from build123d import *

# Parameters (mm, degrees)
CROQUIS1_W              = 8.5
CROQUIS1_H              = 10
SALIENTE_EXTRUIR1_DEPTH = 3.3
CROQUIS2_R              = 0.466725864
CORTAR_EXTRUIR1_DEPTH   = 0.1
CORTAR_EXTRUIR2_DEPTH   = 3
CORTAR_EXTRUIR3_DEPTH   = 3
CHAFL_N1_SIZE           = 0.6
REDONDEO1_R             = 0.3
CROQUIS5_W              = 8.5
CROQUIS5_H              = 0.8
SALIENTE_EXTRUIR2_DEPTH = 5.8
CROQUIS6_R              = 1.750484279
CORTAR_EXTRUIR4_DEPTH   = 5.8
CROQUIS7_W              = 1.22
CROQUIS7_H              = 0.3917794
SALIENTE_EXTRUIR3_DEPTH = 5.3
CROQUIS8_W              = 1.22
CROQUIS8_H              = 0.3917794
SALIENTE_EXTRUIR4_DEPTH = 5.3
CROQUIS9_W              = 0.675717965
CROQUIS9_H              = 1
CROQUIS9_W_2            = 0.619737604
CROQUIS9_W_3            = 0.713804918
SALIENTE_EXTRUIR5_DEPTH = 2.3
CHAFL_N2_SIZE           = 0.3
CHAFL_N3_SIZE           = 0.3
CHAFL_N4_SIZE           = 0.3
CHAFL_N5_SIZE           = 0.3
CHAFL_N6_SIZE           = 0.3
CHAFL_N7_SIZE           = 0.3
CHAFL_N8_SIZE           = 1.29
CHAFL_N9_SIZE           = 1.29


with BuildPart() as part:
    # Croquis1 → Saliente-Extruir1 (new body)
    with BuildSketch(Plane.XY):
        Rectangle(CROQUIS1_W, CROQUIS1_H)
    extrude(amount=SALIENTE_EXTRUIR1_DEPTH)

    # Croquis2 → Cortar-Extruir1 (cut)
    with BuildSketch(Plane.XY.offset(3.3)):
        with Locations((-3.215855375, -4.280210789)):
            Circle(CROQUIS2_R)
    extrude(amount=-CORTAR_EXTRUIR1_DEPTH, mode=Mode.SUBTRACT)

    # Croquis3 → Cortar-Extruir2 (cut)
    with BuildSketch(Plane.XY.offset(3.3)):
        with BuildLine():
            Line((-4.25, 0.746438526), (-4.25, -0.746438526))
            ThreePointArc((-4.25, -0.746438526), (-3.503561474, 0), (-4.25, 0.746438526))
        make_face()
    extrude(amount=-CORTAR_EXTRUIR2_DEPTH, mode=Mode.SUBTRACT)

    # Croquis4 → Cortar-Extruir3 (cut)
    with BuildSketch(Plane.XY.offset(3.3)):
        with BuildLine():
            Line((4.25, 0.878718771), (4.25, -0.633055459))
            ThreePointArc((4.25, -0.633055459), (3.494112885, 0.122831656), (4.25, 0.878718771))
        make_face()
    extrude(amount=-CORTAR_EXTRUIR3_DEPTH, mode=Mode.SUBTRACT)

    # Chaflán1
    chafl_n1_edges = [part.edges().sort_by_distance(p)[0] for p in [
        (0, 5, 3.3),
    ]]
    chamfer(chafl_n1_edges, length=CHAFL_N1_SIZE)

    # Redondeo1
    redondeo1_edges = [part.edges().sort_by_distance(p)[0] for p in [
        (4.25, -2.816527729, 3.3),
        (-4.25, -2.873219263, 3.3),
        (-3.503561474, 0, 3.3),
        (4.25, 2.639359386, 3.3),
        (3.494112885, 0.122831656, 3.3),
        (-4.25, 2.573219263, 3.3),
    ]]
    fillet(redondeo1_edges, radius=REDONDEO1_R)

    # Croquis5 → Saliente-Extruir2 (add)
    with BuildSketch(Plane(origin=(0, 5, 0), x_dir=(1, 0, 0), z_dir=(0, 1, 0))):
        with Locations((0, -0.4)):
            Rectangle(CROQUIS5_W, CROQUIS5_H)
    extrude(amount=SALIENTE_EXTRUIR2_DEPTH)

    # Croquis6 → Cortar-Extruir4 (cut)
    with BuildSketch(Plane.XY.offset(0.8)):
        with Locations((0, 8.041970686)):
            Circle(CROQUIS6_R)
    extrude(amount=-CORTAR_EXTRUIR4_DEPTH, mode=Mode.SUBTRACT)

    # Croquis7 → Saliente-Extruir3 (add)
    with BuildSketch(Plane.XZ.offset(5)):
        with Locations((0, 2.138324213)):
            Rectangle(CROQUIS7_W, CROQUIS7_H)
    extrude(amount=SALIENTE_EXTRUIR3_DEPTH)

    # Croquis8 → Saliente-Extruir4 (add)
    with BuildSketch(Plane.XZ.offset(5)):
        with Locations((2.43, 2.138324213)):
            Rectangle(CROQUIS8_W, CROQUIS8_H)
        with Locations((-2.43, 2.138324213)):
            Rectangle(CROQUIS8_W, CROQUIS8_H)
    extrude(amount=SALIENTE_EXTRUIR4_DEPTH)

    # Croquis9 → Saliente-Extruir5 (add)
    with BuildSketch(Plane(origin=(0, 0, 1.942434513), x_dir=(-1, 0, 0), z_dir=(0, 0, -1))):
        with Locations((-0.032858983, -9.8)):
            Rectangle(CROQUIS9_W, CROQUIS9_H)
        with Locations((2.407034508, -9.8)):
            Rectangle(CROQUIS9_W_2, CROQUIS9_H)
        with Locations((-2.448498949, -9.8)):
            Rectangle(CROQUIS9_W_3, CROQUIS9_H)
    extrude(amount=SALIENTE_EXTRUIR5_DEPTH)

    # Chaflán2
    chafl_n2_edges = [part.edges().sort_by_distance(p)[0] for p in [
        (3.04, -10.3, 2.138324213),
    ]]
    chamfer(chafl_n2_edges, length=CHAFL_N2_SIZE)

    # Chaflán3
    chafl_n3_edges = [part.edges().sort_by_distance(p)[0] for p in [
        (1.82, -10.3, 2.138324213),
    ]]
    chamfer(chafl_n3_edges, length=CHAFL_N3_SIZE)

    # Chaflán4
    chafl_n4_edges = [part.edges().sort_by_distance(p)[0] for p in [
        (-0.61, -10.3, 2.138324213),
    ]]
    chamfer(chafl_n4_edges, length=CHAFL_N4_SIZE)

    # Chaflán5
    chafl_n5_edges = [part.edges().sort_by_distance(p)[0] for p in [
        (-3.04, -10.3, 2.138324213),
    ]]
    chamfer(chafl_n5_edges, length=CHAFL_N5_SIZE)

    # Chaflán6
    chafl_n6_edges = [part.edges().sort_by_distance(p)[0] for p in [
        (-1.82, -10.3, 2.138324213),
    ]]
    chamfer(chafl_n6_edges, length=CHAFL_N6_SIZE)

    # Chaflán7
    chafl_n7_edges = [part.edges().sort_by_distance(p)[0] for p in [
        (0.61, -10.3, 2.138324213),
    ]]
    chamfer(chafl_n7_edges, length=CHAFL_N7_SIZE)

    # Chaflán8
    chafl_n8_edges = [part.edges().sort_by_distance(p)[0] for p in [
        (4.25, 10.8, 0.4),
    ]]
    chamfer(chafl_n8_edges, length=CHAFL_N8_SIZE)

    # Chaflán9
    chafl_n9_edges = [part.edges().sort_by_distance(p)[0] for p in [
        (-4.25, 10.8, 0.4),
    ]]
    chamfer(chafl_n9_edges, length=CHAFL_N9_SIZE)


solid = part.part
Source: CAD feature listing. Evaluate the final solid. Frame: model axes, mm. A direction names the side the tool comes from. Round coordinates to 2 decimals unless told otherwise and drop trailing zeros. Loops run counter-clockwise (first coordinate to the right, second up) from the corner with the lowest first, then second, coordinate; pieces in that order, holes last.
Q1. Section B-B, the plane x = 0. Return loops of the section in (y, z).
Q2. Access query for faces 1 (the face through (0, 6, 0.8)), 2 (the face through (0.371, -10, 1)), 3 (the face through (-3.504, -0.016, 1.669)). Directions: +Z, -Z, +X, -X, +Y, -Y. A direction counts if a zero-diameter tool reaches every point of the face in a straight line with its end or side. Return the directions, or none.
Q3. First-contact query: P1, Ø1, axis at x = 0, y = -8, coming from the -Z side; P2, Ø2.5, axis at x = 1, y = 0, coming from the -Z side; P3, Ø4, axis at x = 0, y = 8.04, coming from the +Z side. Flat tips, straight axial feed; report the tip coordinate or a pass-through.
Q4. Mould query, pull axis Y, two halves, no side actions, for faces 4 (the face through (-2, -8, 1.942)), 5 (the face through (0, 5, 2)), 6 (the face through (2.092, -10, 1)). Classes: pulls with the +Y half, pulls with the -Y half, needs draft (parallel to the pull), parting line crosses it, or undercut.
Q5. Section C-C, the plane y = 1.75. Return loops of the section in (x, z), plus the area to 3 significant figures.
Q6. Section A-A, the plane y = -6. Return loops of the section in (x, z), plus the area to 3 significant figures.
Q7. Section D-D, the plane x = -1.5. Return loops of the section in (y, z).
Q8. Ray query, line 1 (Y direction, x = 0, z = 0.4); line 2 (X direction, y = -5.75, z = 2.2); line 3 (Y direction, x = -1.75, z = 1.05). Return the intervals inside material, ascending.
Solutions:
1. outline: (-10.3, -0.36) - (-9.3, -0.36) - (-9.3, 1.94) - (-5, 1.94) - (-5, 0) - (6.29, 0) - (6.29, 0.8) - (5, 0.8) - (5, 2.7) - (4.4, 3.3) - (-5, 3.3) - (-5, 2.33) - (-10.3, 2.33) - close; (9.79, 0) - (10.8, 0) - (10.8, 0.8) - (9.79, 0.8) - close
2. face 1: +Z, +X, -X, +Y
2. face 2: -Z, -Y
2. face 3: +Z, -X
3. P1: stops at z = 1.94
3. P2: stops at z = 0
3. P3: stops at z = 0.8
4. face 4: undercut
4. face 5: pulls with the +Y half
4. face 6: needs draft
5. outline: (-4.25, 0) - (4.25, 0) - (4.25, 3) arc R0.3 ccw to (3.95, 3.3) - (-3.95, 3.3) arc R0.3 ccw to (-4.25, 3) - close
5. area: 28.0 mm2
6. outline: (-3.04, 1.94) - (-1.82, 1.94) - (-1.82, 2.33) - (-3.04, 2.33) - close; (-0.61, 1.94) - (0.61, 1.94) - (0.61, 2.33) - (-0.61, 2.33) - close; (1.82, 1.94) - (3.04, 1.94) - (3.04, 2.33) - (1.82, 2.33) - close
6. area: 1.43 mm2
7. outline: (-5, 0) - (7.14, 0) - (7.14, 0.8) - (5, 0.8) - (5, 2.7) - (4.4, 3.3) - (-5, 3.3) - close; (8.94, 0) - (10.8, 0) - (10.8, 0.8) - (8.94, 0.8) - close
8. line 1: y = -10.3 to -9.3, -5 to 6.29, 9.79 to 10.8
8. line 2: x = -3.04 to -1.82, -0.61 to 0.61, 1.82 to 3.04
8. line 3: y = -5 to 5
